Part print with two shaded views. Sizes in mm from the minimum x, y, z corner. A direction names the side the tool comes from. Round coordinates to 2 decimals unless told otherwise and drop trailing zeros. Order: outer loops, then holes, each group sorted by start corner. A loop starts at its lowest first (then second) coordinate and runs counter-clockwise, first axis right, second up. Notation, with made-up numbers: M 29,-20 L 78,-20 A12 cw 78,-8 Z; hole C 39,44.25 d6. An arc over 180 degrees is marked long. Return JSON: item names as keys, results as strings. Group by question number.
Item 1: Probe line 1 along Y through (x, z) = (5.75, 1); line 2 along Y through (x, z) = (7, 6.5); line 3 along Y through (x, z) = (4.5, 6). List the from-to ranges inside material, lowest first.
Item 2: Slice it at C-C on y = 15.75. Write the cut outline in (x, z), then the cut area to 3 significant figures.
Item 3: Slice it at B-B on z = 2. Write the cut outline in (x, y).
Item 4: Slice it at A-A on x = 5. Write the cut outline in (y, z).
Item 5: Pull direction Y, two halves, no side cores. Call the marked faces 1, 2, 3 and 4: pulls with the +Y half, pulls with the -Y half, needs draft (parallel to the pull), parting line crosses it, or undercut.
Item 6: Pin check, flat tips, straight feed: pin 1 Ø4 at (y, z) = (3, 11) entering from +X; pin 2 Ø2 at (x, z) = (5.5, 10) entering from -Y; pin 3 Ø5 at (y, z) = (3.5, 8) entering from +X; pin 4 Ø4 at (x, z) = (7, 8) entering from +Y. Stop position of each tip, or through.
Item 7: Slice it at D-D on x = 9. Write the cut outline in (y, z).
Item 8: Which spindle directions (+Z, -Z, +X, -X, +Y, -Y) get a long thin tool onto all of the face, cutting with end or side? Do the marked faces 5 and 6. Say none if no direction does.
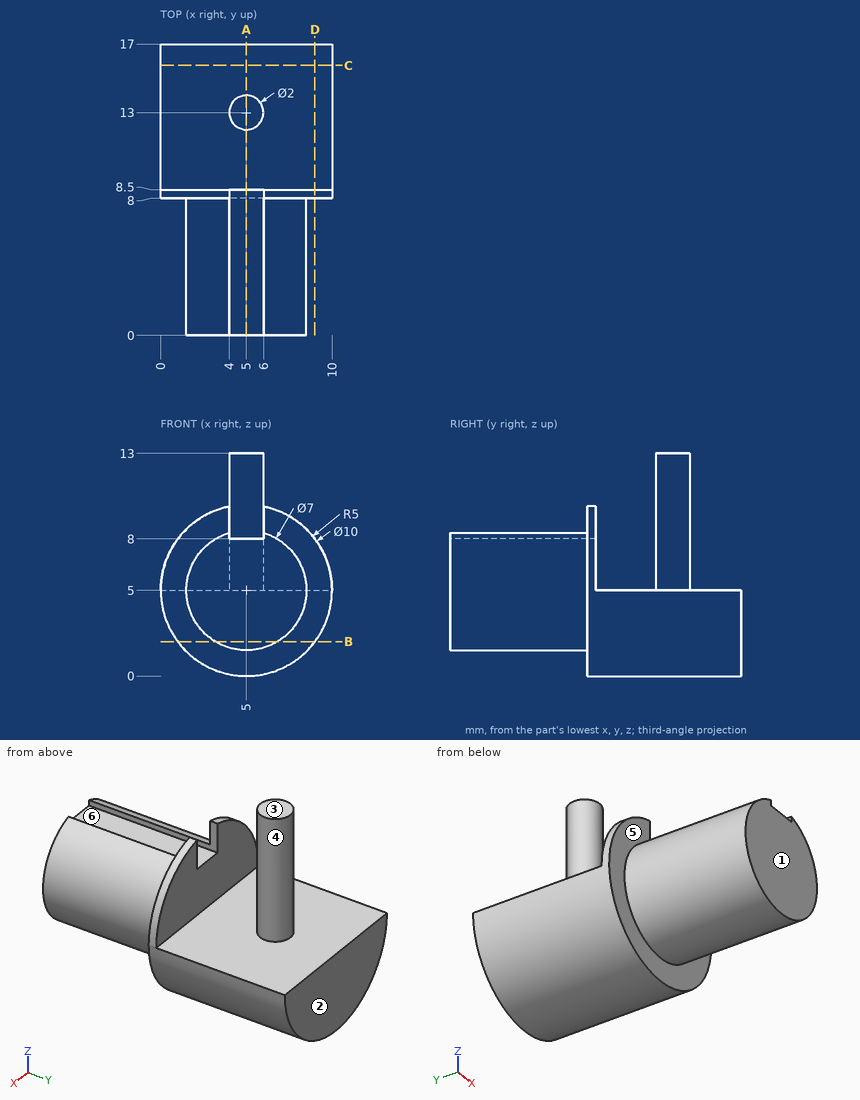
Output values:
{
 "1": {"line 1": "8 to 17", "line 2": "0 to 8.5", "line 3": "0 to 8.5, 12.13 to 13.87"},
 "2": {"outline": "M 0,5 A5 ccw 10,5 Z", "area": "39.3 mm²"},
 "3": {"outline": "M 1,8 L 3.2,8 L 3.2,0 L 6.8,0 L 6.8,8 L 9,8 L 9,17 L 1,17 Z"},
 "4": {"outline": "M 0,1.5 L 8,1.5 L 8,0 L 17,0 L 17,5 L 14,5 L 14,13 L 12,13 L 12,5 L 8.5,5 L 8.5,8 L 0,8 Z"},
 "5": {"face 1": "pulls with the -Y half", "face 2": "pulls with the +Y half", "face 3": "needs draft", "face 4": "undercut"},
 "6": {"pin 1": "through", "pin 2": "y = 8", "pin 3": "x = 8.46", "pin 4": "y = 14"},
 "7": {"outline": "M 8,2 L 17,2 L 17,5 L 8.5,5 L 8.5,8 L 8,8 Z"},
 "8": {"face 5": "-Y", "face 6": "+Z, -Y"}
}
